```python
from build123d import *

# Parameters (mm, degrees)
F0_W     = 200
F0_H     = 150
F1_DEPTH = 25
F2_R     = 9.968788
F3_DEPTH = 15
F5_DEPTH = 15


with BuildPart() as f1:
    # F0 (on Top) → F1 (new body)
    with BuildSketch(Plane.XY):
        with Locations((24.923838, -0.264797)):
            Rectangle(F0_W, F0_H)
    extrude(amount=F1_DEPTH)

    # F2 (on face) → F3 (cut)
    with BuildSketch(Plane.XY.offset(25)):
        with Locations((24.923838, 54.140884)):
            Circle(F2_R)
    extrude(amount=-F3_DEPTH, mode=Mode.SUBTRACT)

    # F4 (on face) → F5 (cut)
    with BuildSketch(Plane.XY.offset(25)):
        with BuildLine():
            Line((-10.076162, 45.415138), (-45.076162, 45.415138))
            ThreePointArc((-45.076162, 45.415138), (-48.611696, 43.950672), (-50.076162, 40.415138))
            Line((-50.076162, 40.415138), (-50.076162, -45.985725))
            ThreePointArc((-50.076162, -45.985725), (-48.611696, -49.521259), (-45.076162, -50.985725))
            Line((-45.076162, -50.985725), (-10.076162, -50.985725))
            ThreePointArc((-10.076162, -50.985725), (-6.540628, -49.521259), (-5.076162, -45.985725))
            Line((-5.076162, -45.985725), (-5.076162, 40.415138))
            ThreePointArc((-5.076162, 40.415138), (-6.540628, 43.950672), (-10.076162, 45.415138))
        make_face()
        with BuildLine():
            Line((94.923838, 45.415138), (59.923838, 45.415138))
            ThreePointArc((59.923838, 45.415138), (56.388304, 43.950672), (54.923838, 40.415138))
            Line((54.923838, 40.415138), (54.923838, -45.985725))
            ThreePointArc((54.923838, -45.985725), (56.388304, -49.521259), (59.923838, -50.985725))
            Line((59.923838, -50.985725), (94.923838, -50.985725))
            ThreePointArc((94.923838, -50.985725), (98.459372, -49.521259), (99.923838, -45.985725))
            Line((99.923838, -45.985725), (99.923838, 40.415138))
            ThreePointArc((99.923838, 40.415138), (98.459372, 43.950672), (94.923838, 45.415138))
        make_face()
    extrude(amount=-F5_DEPTH, mode=Mode.SUBTRACT)


solid = f1.part
```
Geometry check sheet. Reference: the model listing, model coordinates, mm. A direction names the side the tool comes from. Coordinates: 2 decimals unless noted, no trailing zeros. Loops run counter-clockwise (first coordinate to the right, second up) from the corner with the lowest first, then second, coordinate; pieces in that order, holes last. Notation, with made-up numbers: (-36.75, 51) -> (12.25, 51) arc R32 ccw to (12.25, 77) -> close; hole circle Ø2 at (41, 55.25). An arc over 180 degrees is marked (long way). Put each result on its own line as item: value.
1) Release check for a two-part mould opening along X. For faces 3 (the flat face through (124.924, -1, 12)), 4 (the flat face through (24, -75.265, 12)), 5 (the cylindrical face through (56.43, 43.99, 17.6)) record: released by +X, released by -X, zero draft, split by the parting line, or undercut.
Result set:
face 3: released by +X
face 4: zero draft
face 5: undercut
2) Cross-section at C-C on y = -30.5. Record the boundary of the cut face in (x, z), plus the area to 3 significant figures.
Result set:
outline: (-75.08, 0) -> (124.92, 0) -> (124.92, 25) -> (99.92, 25) -> (99.92, 10) -> (54.92, 10) -> (54.92, 25) -> (-5.08, 25) -> (-5.08, 10) -> (-50.08, 10) -> (-50.08, 25) -> (-75.08, 25) -> close
area: 3,650 mm^2
3) Gauge pin test, flat end, axial feed: pin 1 Ø6 at (x, y) = (24.5, 54) entering from +Z. Record the tip position at first contact, or that the pin passes through.
Result set:
pin 1: stops at z = 10
4) Cross-section at B-B on x = 71. Record the boundary of the cut face in (y, z).
Result set:
outline: (-75.26, 0) -> (74.74, 0) -> (74.74, 25) -> (45.42, 25) -> (45.42, 10) -> (-50.99, 10) -> (-50.99, 25) -> (-75.26, 25) -> close
5) Cross-section at D-D on x = -8. Record the boundary of the cut face in (y, z).
Result set:
outline: (-75.26, 0) -> (74.74, 0) -> (74.74, 25) -> (44.96, 25) -> (44.96, 10) -> (-50.53, 10) -> (-50.53, 25) -> (-75.26, 25) -> close
6) Thickness scan on line 1 (X direction, y = 38.5, z = 13); line 2 (Y direction, x = -39, z = 15.25); line 3 (Y direction, x = 31.5, z = 18.5). Record the ranges inside material, lowest first.
Result set:
line 1: x = -75.08 to -50.08, -5.08 to 54.92, 99.92 to 124.92
line 2: y = -75.26 to -50.99, 45.42 to 74.74
line 3: y = -75.26 to 46.65, 61.63 to 74.74
7) Tool access check on faces 1 (the flat face through (24, 1, 0)), 2 (the flat face through (-5.076, -3, 18)). Record the directions out of +Z, -Z, +X, -X, +Y, -Y that give a thin tool (end or side, any length) a straight path to the whole face; none if there is none.
Result set:
face 1: -Z, +X, -X, +Y, -Y
face 2: +Z
8) Cross-section at A-A on z = 22.25. Record the boundary of the cut face in (x, y).
Result set:
outline: (-75.08, -75.26) -> (124.92, -75.26) -> (124.92, 74.74) -> (-75.08, 74.74) -> close; hole (-50.08, -45.99) arc R5 ccw to (-45.08, -50.99) -> (-10.08, -50.99) arc R5 ccw to (-5.08, -45.99) -> (-5.08, 40.42) arc R5 ccw to (-10.08, 45.42) -> (-45.08, 45.42) arc R5 ccw to (-50.08, 40.42) -> close; hole circle Ø19.94 at (24.92, 54.14); hole (54.92, -45.99) arc R5 ccw to (59.92, -50.99) -> (94.92, -50.99) arc R5 ccw to (99.92, -45.99) -> (99.92, 40.42) arc R5 ccw to (94.92, 45.42) -> (59.92, 45.42) arc R5 ccw to (54.92, 40.42) -> close
